Geometry: see drawing. Coordinates: mm, zero at the bounding-box minimum. A direction names the side the tool comes from. Round coordinates to 2 decimals unless told otherwise and drop trailing zeros. Loops run counter-clockwise (first coordinate to the right, second up) from the corner with the lowest first, then second, coordinate; pieces in that order, holes last. Notation, with made-up numbers: M 86,7.25 L 120,7.25 A20 ccw 120,21.25 Z; hole C 17.5,10 d2. An arc over 180 degrees is marked long. Answer as a JSON object with one key per item and string values.
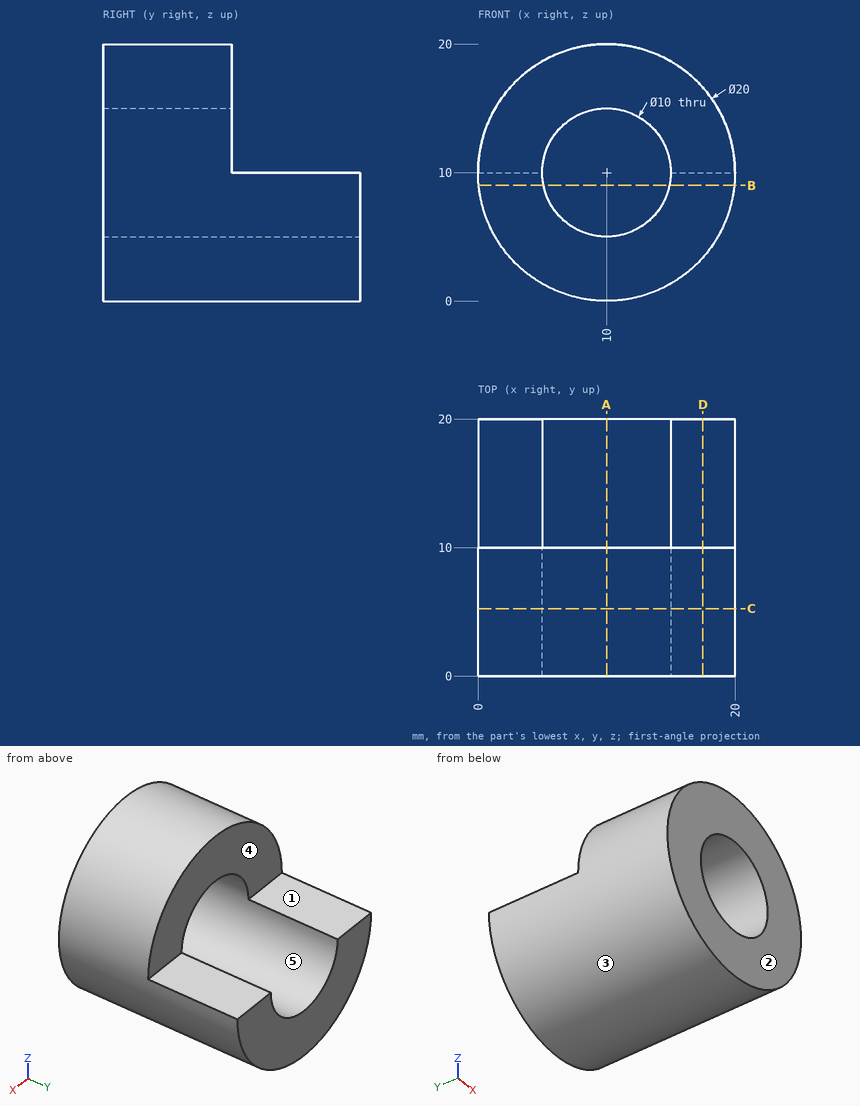
1) Section query B-B (z = 9). Return the cut outline in (x, y), and give its area (3 significant figures).
Results:
{"outline": "M 0.05,0 L 5.1,0 L 5.1,20 L 0.05,20 Z; M 14.9,0 L 19.95,0 L 19.95,20 L 14.9,20 Z", "area": "202 mm2"}
2) Section query A-A (x = 10). Return the cut outline in (y, z), and give its area (3 significant figures).
Results:
{"outline": "M 0,0 L 20,0 L 20,5 L 0,5 Z; M 0,15 L 10,15 L 10,20 L 0,20 Z", "area": "150 mm2"}
3) Pin query (flat end, axial travel): P1, Ø8, axis at x = 9.5, z = 16.5, coming from the +Y side; P2, Ø1.5, axis at y = 12, z = 3.5, coming from the -X side; P3, Ø1.5, axis at y = 10, z = 13, coming from the +X side; P4, Ø4, axis at x = 10.5, y = 13.5, coming from the -Z side. Return the tip coordinate at first contact, or that it passes through.
Results:
{"P1": "y = 10", "P2": "x = 1.82", "P3": "x = 19.74", "P4": "z = 0"}
4) Section query D-D (x = 17.5). Return the cut outline in (y, z), and give its area (3 significant figures).
Results:
{"outline": "M 0,3.39 L 20,3.39 L 20,10 L 10,10 L 10,16.61 L 0,16.61 Z", "area": "198 mm2"}
5) Section query C-C (y = 5.25). Return the cut outline in (x, z), and give its area (3 significant figures).
Results:
{"outline": "C 10,10 d20; hole C 10,10 d10", "area": "236 mm2"}
6) Ray query, line 1 (Z direction, x = 10, y = 6.5); line 2 (Y direction, x = 8.75, z = 15.5). Return the intervals inside material, ascending.
Results:
{"line 1": "0 to 5, 15 to 20", "line 2": "0 to 10"}
7) Pull-direction query (X, two-part tool) for the marked faces 3, 4 and 5; classes: +X half, -X half, draft (parallel to the pull), parting line (faces both ways), or undercut.
Results:
{"face 3": "parting line", "face 4": "draft", "face 5": "undercut"}
8) Reachability of the marked faces 1 and 2 from +Z, -Z, +X, -X, +Y, -Y: full face, straight path, thin tool, end or side. Return the list, or none.
Results:
{"face 1": "+Z, +X, -X, +Y", "face 2": "+Z, -Z, +X, -X, -Y"}
